Here's how the part is built. I have some questions about the finished solid (model axes, mm). Round coordinates to 2 decimals unless told otherwise and drop trailing zeros. Write each loop counter-clockwise with the first axis right and the second up, starting at its lowest first coordinate (ties: lowest second). Pieces come first, ordered by that corner, then holes. Notation, with made-up numbers: (8, -5) -> (26, -5) arc R20 ccw to (26, 28) -> close; hole circle Ø11 at (53.5, 35). An arc over 180 degrees is marked (long way). Answer in a Markdown table with one row per item. Add a question column.
from build123d import *

# Parameters (mm, degrees)
F0_W     = 15.5
F0_H     = 15.5
F0_R     = 3
F1_DEPTH = 3


with BuildPart() as f1:
    # F0 (on Front) → F1 (new body)
    with BuildSketch(Plane.XZ):
        with BuildLine():
            ThreePointArc((7.75, 7.75), (0, 15.5), (-7.75, 7.75))
            Line((-7.75, 7.75), (7.75, 7.75))
        make_face()
        Rectangle(F0_W, F0_H)
        Circle(F0_R, mode=Mode.SUBTRACT)
        with BuildLine():
            Line((7.75, -7.75), (-7.75, -7.75))
            ThreePointArc((-7.75, -7.75), (0, -15.5), (7.75, -7.75))
        make_face()
    extrude(amount=F1_DEPTH)


solid = f1.part
Item 1: If we section it at A-A on x = 0: Please give me the cut outline in (y, z).
Item 2: I need wall thicknesses on line 1 along Z through (x, y) = (0, -1.75); line 2 along X through (y, z) = (-0.25, 2.5); line 3 along X through (y, z) = (-0.85, 1). Which ranges of each line are inside material? Lowest first, please. Write a range as from..to.
Item 3: If we mould it in two halves opening along Z, with no side actions, what happens to faces 1 (the flat face through (-0.1, -3, -3.2)), 2 (the cylindrical face through (-0.17, -1.48, -15.5)), 3 (the cylindrical face through (-3, -1, 0)), 4 (the cylindrical face through (0.17, -1.48, 15.5))? For each: pulls with the +Z half, pulls with the -Z half, needs draft (parallel to the pull), parting line crosses it, or undercut.
Item 4: If we section it at B-B on z = 0: Please give me the cut outline in (x, y), then the cut area to 3 significant figures.
Item 5: If we section it at D-D on x = -4.5: Please give me the cut outline in (y, z), then the cut area to 3 significant figures.
Item 6: If we section it at C-C on y = -1: Please give me the cut outline in (x, z).
Item 7: For P1, Ø1.5, axis at x = 3.5, y = -2, coming from the +Z side; P2, Ø1, axis at x = 4, y = -0.5, coming from the -Z side; P3, Ø1.5, axis at y = -1.5, z = -9, coming from the +X side, each with a flat end and sliding along its axis, tell me the tip position at first contact or that it passes through.
Results list:
| question | item | result |
|---|---|---|
| 1 | outline | (-3, -15.5) -> (0, -15.5) -> (0, -3) -> (-3, -3) -> close; (-3, 3) -> (0, 3) -> (0, 15.5) -> (-3, 15.5) -> close |
| 2 | line 1 | -15.5..-3, 3..15.5 |
| 2 | line 2 | -7.75..-1.66, 1.66..7.75 |
| 2 | line 3 | -7.75..-2.83, 2.83..7.75 |
| 3 | face 1 | needs draft |
| 3 | face 2 | pulls with the -Z half |
| 3 | face 3 | undercut |
| 3 | face 4 | pulls with the +Z half |
| 4 | outline | (-7.75, -3) -> (-3, -3) -> (-3, 0) -> (-7.75, 0) -> close; (3, -3) -> (7.75, -3) -> (7.75, 0) -> (3, 0) -> close |
| 4 | area | 28.5 mm² |
| 5 | outline | (-3, -14.06) -> (0, -14.06) -> (0, 14.06) -> (-3, 14.06) -> close |
| 5 | area | 84.4 mm² |
| 6 | outline | (-7.75, -7.75) arc R7.75 ccw to (7.75, -7.75) -> (7.75, 7.75) arc R7.75 ccw to (-7.75, 7.75) -> close; hole circle Ø6 at (0, 0) |
| 7 | P1 | z = 15 |
| 7 | P2 | z = -14.66 |
| 7 | P3 | x = 7.73 |
